Geometry check sheet. Reference: drawing and pictorial views, mm from the part's lowest x, y, z. A direction names the side the tool comes from. Give positions to 0.01 mm unless a question says otherwise; leave off trailing zeros. Write each loop counter-clockwise with the first axis right and the second up, starting at its lowest first coordinate (ties: lowest second). Pieces come first, ordered by that corner, then holes. Notation, with made-up numbers: (53, 38.25) -> (109, 38.25) arc R34 ccw to (109, 73.25) -> close; hole circle Ø8 at (-25, -2). An arc over 180 degrees is marked (long way). Write each question's results on one line, items separated by ' | '. Start each with the question number.
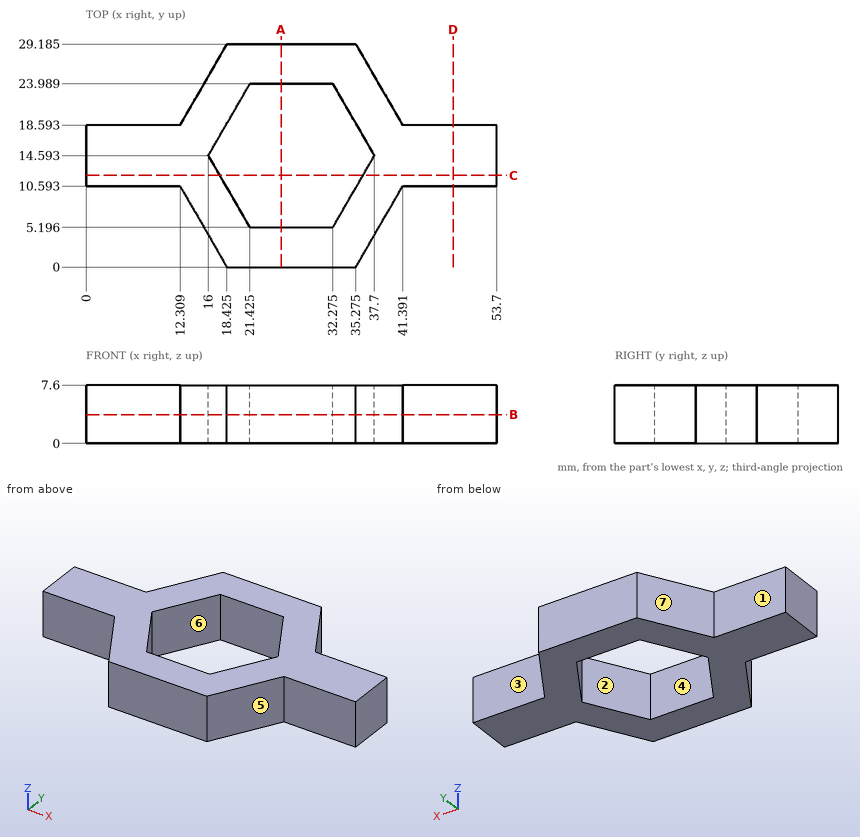
Item 1: Depth check by flat-ended pin: pin 1 Ø4 at (x, z) = (15, 5) entering from -Y; pin 2 Ø2.5 at (x, z) = (47, 2) entering from -Y; pin 3 Ø2.5 at (x, z) = (46, 4) entering from +Y; pin 4 Ø3 at (y, z) = (18, 5.5) entering from -X. Enter the tip coordinate at first touch or a pass-through.
Item 2: Section check B-B on z = 3.75. Record the boundary of the cut face in (x, y) (1 decimal).
Item 3: Mould release check, pull along Y, two halves, no side actions. Record for the marked faces 4, 5, 6 and 7: pulls with the +Y half, pulls with the -Y half, needs draft (parallel to the pull), parting line crosses it, or undercut.
Item 4: Thickness scan on probe 1 along Y at (x, z) = (29, 0.5) (1 decimal); probe 2 along X at (y, z) = (14, 5.5); probe 3 along Y at (x, z) = (11, 2.25). Record the ranges inside material, lowest first. Write a range as from..to.
Item 5: Set-up check for the marked faces 1, 2 and 3: record each of +Z, -Z, +X, -X, +Y, -Y from which the full face is reachable in a straight line by a thin tool's end or side.
Item 6: Section check A-A on x = 25.5. Record the boundary of the cut face in (y, z) (1 decimal).
Item 7: Section check D-D on x = 48. Record the boundary of the cut face in (y, z).
Item 8: Section check C-C on y = 12. Record the boundary of the cut face in (x, z), then the cut area to 3 significant figures.
Check sheet entries:
1) pin 1: stops at y = 2.47 | pin 2: stops at y = 10.59 | pin 3: stops at y = 18.59 | pin 4: stops at x = 0
2) outline: (0, 10.6) -> (12.3, 10.6) -> (18.4, 0) -> (35.3, 0) -> (41.4, 10.6) -> (53.7, 10.6) -> (53.7, 18.6) -> (41.4, 18.6) -> (35.3, 29.2) -> (18.4, 29.2) -> (12.3, 18.6) -> (0, 18.6) -> close; hole (16, 14.6) -> (21.4, 5.2) -> (32.3, 5.2) -> (37.7, 14.6) -> (32.3, 24) -> (21.4, 24) -> close
3) face 4: undercut | face 5: pulls with the -Y half | face 6: undercut | face 7: pulls with the +Y half
4) probe 1: y = 0..5.2, 24..29.2 | probe 2: x = 0..16.34, 37.36..53.7 | probe 3: y = 10.59..18.59
5) face 1: +Z, -Z, -X, +Y | face 2: +Z, -Z | face 3: +Z, -Z, +X, +Y
6) outline: (0, 0) -> (5.2, 0) -> (5.2, 7.6) -> (0, 7.6) -> close; (24, 0) -> (29.2, 0) -> (29.2, 7.6) -> (24, 7.6) -> close
7) outline: (10.59, 0) -> (18.59, 0) -> (18.59, 7.6) -> (10.59, 7.6) -> close
8) outline: (0, 0) -> (17.5, 0) -> (17.5, 7.6) -> (0, 7.6) -> close; (36.2, 0) -> (53.7, 0) -> (53.7, 7.6) -> (36.2, 7.6) -> close | area: 266 mm^2
